Autodesk Inventor part; units mm, degrees
ref_plane "YZ Plane" through (0, 0, 0) normal (1, 0, 0) x (0, 1, 0)
ref_plane "XZ Plane" through (0, 0, 0) normal (0, 1, 0) x (-1, 0, 0)
ref_plane "XY Plane" through (0, 0, 0) normal (0, 0, 1) x (1, 0, 0)
sketch "Sketch1" plane through (0, 0, 0) normal (0, 0, 1) x (1, 0, 0)
  line L0 (-21, 21) -> (21, 21)
  line L1 (21, 21) -> (21, -21)
  line L2 (21, -21) -> (-21, -21)
  line L3 (-21, -21) -> (-21, 21)
  point P0 (0, 0)
  point P1 (0, 0)
  dimension "d0" = 42
extrude "Extrusion1" add sketch "Sketch1" along normal mid plane 48
sketch "Sketch2" plane through (0, 0, 24) normal (0, 0, 1) x (1, 0, 0)
  circle A0 centre (0, 0) radius 11
  dimension "d3" = 22
extrude "Extrusion2" add sketch "Sketch2" along normal blind 2
sketch "Sketch3" plane through (0, 0, 26) normal (0, 0, 1) x (1, 0, 0)
  circle A0 centre (0, 0) radius 11
  circle A1 centre (0, 0) radius 2.5
  dimension "d7" = 5
extrude "Extrusion3" add sketch "Sketch3" along normal blind 22 contours A1
sketch "Sketch4" plane through (0, 0, 48) normal (0, 0, 1) x (1, 0, 0)
  circle A0 centre (0, 0) radius 2.5
  line L0 (-1.5, 2) -> (1.5, 2)
  dimension "d11" = 2
extrude "Extrusion4" cut sketch "Sketch4" against normal blind 15 contours L0 A0 picked at (-0.3466, 2.0912)
sketch "Sketch5" plane through (0, 0, 24) normal (0, 0, 1) x (1, 0, 0)
  circle A0 centre (0, 0) radius 11
  line L0 (-15.5, 15.5) -> (15.5, 15.5)
  line L1 (15.5, 15.5) -> (15.5, -15.5)
  line L2 (15.5, -15.5) -> (-15.5, -15.5)
  line L3 (-15.5, -15.5) -> (-15.5, 15.5)
  dimension "d14" = 31
hole "Hole1" at (-15.5, 15.5, 24) at (15.5, 15.5, 24) at (15.5, -15.5, 24) at (-15.5, -15.5, 24) direction (0, 0, -1) diameter 2.459 end through all
chamfer "Chamfer1" distance 5 angle 45 4 edges at (21, 21, 0) (-21, 21, 0) (21, -21, 0) (-21, -21, 0)
sketch "Sketch6" plane through (0, 0, 0) normal (0, 0, 1) x (1, 0, 0)
  line L0 (-21, 16) -> (-16, 21)
  line L1 (-16, 21) -> (16, 21)
  line L2 (16, 21) -> (21, 16)
  line L3 (21, 16) -> (21, -16)
  line L4 (21, -16) -> (16, -21)
  line L5 (16, -21) -> (-16, -21)
  line L6 (-16, -21) -> (-21, -16)
  line L7 (-21, -16) -> (-21, 16)
  circle A0 centre (15.5, -15.5) radius 1.2295
  circle A1 centre (-15.5, 15.5) radius 1.2295
  circle A2 centre (15.5, 15.5) radius 1.2295
  circle A3 centre (-15.5, -15.5) radius 1.2295
  line L8 (-21, 13.1716) -> (-13.1716, 21)
  point P0 (0, 0)
  dimension "d25" = 2
extrude "Extrusion5" cut sketch "Sketch6" along normal mid plane 30 contours L0 L1 L8 L7
pattern_circular "Circular Pattern1" count 4 over 360 about axis through (0, 0, 26) along (0, 0, 1) of "Extrusion5"
sketch "Sketch7" plane through (-16, -21, 24) normal (0, -1, 0) x (1, 0, 0)
  line L0 (-5, -39) -> (-5, -9)
  line L1 (-5, -39) -> (2.8284, -39)
  line L2 (2.8284, -9) -> (2.8284, -39)
  line L3 (2.8284, -9) -> (-5, -9)
  line L4 (29.1716, -39) -> (29.1716, -9)
  line L5 (29.1716, -39) -> (37, -39)
  line L6 (37, -9) -> (37, -39)
  line L7 (37, -9) -> (29.1716, -9)
  line L8 (-5, -9) -> (37, -9)
  line L9 (37, -9) -> (37, -39)
  line L10 (37, -39) -> (-5, -39)
  line L11 (-5, -39) -> (-5, -9)
  point P0 (16, -24)
extrude "Extrusion6" cut sketch "Sketch7" against normal blind 0.1
pattern_circular "Circular Pattern2" count 4 over 360 about axis through (0, 0, 26) along (0, 0, 1) of "Extrusion6"
properties part number "stepper"
Could you check a few things on this model? Use its own coordinates, in mm. A direction names the side the tool comes from. Round coordinates to 2 decimals unless told otherwise and drop trailing zeros. Write each loop counter-clockwise with the first axis right and the second up, starting at its lowest first coordinate (ties: lowest second). Pieces come first, ordered by that corner, then holes.
(1) Suppose I cut it at D-D on z = -3.5. Write out the boundary of the cut face in (x, y), and give its area (3 significant figures).
Findings below:
outline: (-20.9, -13.27) - (-13.27, -20.9) - (13.27, -20.9) - (20.9, -13.27) - (20.9, 13.27) - (13.27, 20.9) - (-13.27, 20.9) - (-20.9, 13.27) - close; hole circle Ø2.46 at (-15.5, -15.5); hole circle Ø2.46 at (-15.5, 15.5); hole circle Ø2.46 at (15.5, -15.5); hole circle Ø2.46 at (15.5, 15.5)
area: 1,610 mm2
(2) Which directions (+Z, -Z, +X, -X, +Y, -Y) give clear straight access to the entire face, cutting with the end or side of a thin tool? Please do faces 1 (the face through (0, 2, 41)), 2 (the face through (17.14, -17.03, -0.21)), 3 (the face through (-20.9, 0, 0)), 4 (the face through (-17.03, -17.14, -0.21)).
Findings below:
face 1: +Z, +X, -X, +Y
face 2: +X, -Y
face 3: -X, +Y, -Y
face 4: -X, -Y
(3) For pin 1 (12.5 mm diameter, centred on x = 7.5, y = 10.5, fed in from +Z); pin 2 (3 mm diameter, centred on x = -15.5, y = 15.5, fed in from -Z); pin 3 (0.6 mm diameter, centred on x = 0, y = 2.5, fed in from +Z); pin 4 (3 mm diameter, centred on x = 15.5, y = -15.5, fed in from +Z), each with a flat end and sliding along its axis, tell me the tip position at first contact or that it passes through.
Findings below:
pin 1: stops at z = 26
pin 2: stops at z = -24
pin 3: stops at z = 33
pin 4: stops at z = 24
(4) Suppose I cut it at B-B on x = 0. Write out the boundary of the cut face in (y, z), and give its area (3 significant figures).
Findings below:
outline: (-21, -24) - (21, -24) - (21, -15) - (20.9, -15) - (20.9, 15) - (21, 15) - (21, 24) - (11, 24) - (11, 26) - (2.5, 26) - (2.5, 33) - (2, 33) - (2, 48) - (-2.5, 48) - (-2.5, 26) - (-11, 26) - (-11, 24) - (-21, 24) - (-21, 15) - (-20.9, 15) - (-20.9, -15) - (-21, -15) - close
area: 2,160 mm2
(5) Suppose I cut it at C-C on y = 0. Write out the boundary of the cut face in (x, z), and give its area (3 significant figures).
Findings below:
outline: (-21, -24) - (21, -24) - (21, -15) - (20.9, -15) - (20.9, 15) - (21, 15) - (21, 24) - (11, 24) - (11, 26) - (2.5, 26) - (2.5, 48) - (-2.5, 48) - (-2.5, 26) - (-11, 26) - (-11, 24) - (-21, 24) - (-21, 15) - (-20.9, 15) - (-20.9, -15) - (-21, -15) - close
area: 2,160 mm2
(6) Suppose I cut it at A-A on z = 21. Write out the boundary of the cut face in (x, y), and give its area (4 significant figures).
Findings below:
outline: (-21, -16) - (-16, -21) - (16, -21) - (21, -16) - (21, 16) - (16, 21) - (-16, 21) - (-21, 16) - close; hole circle Ø2.46 at (-15.5, -15.5); hole circle Ø2.46 at (-15.5, 15.5); hole circle Ø2.46 at (15.5, -15.5); hole circle Ø2.46 at (15.5, 15.5)
area: 1,695 mm2
(7) Thinking about a two-plate mould opening in Z: for faces 5 (the face through (21, 0, 19)), 6 (the face through (17.2, 17.2, -15)), 7 (the face through (9, -9, 24)), which applies, +Z half, -Z half, draft (parallel to the pull), parting line (faces both ways), or undercut?
Findings below:
face 5: draft
face 6: undercut
face 7: +Z half
(8) If I drill on probe 1 along X at (y, z) = (-15.5, -12.5); probe 2 along Z at (x, y) = (-12.5, 16.5), over which ranges is the centre line in solid material (lowest first)?
Findings below:
probe 1: x = -18.67 to -16.73, -14.27 to 14.27, 16.73 to 18.67
probe 2: z = -24 to 24
